```python
from build123d import *

# Parameters (mm, degrees)
SKETCH1_W           = 34
SKETCH1_H           = 17
SKETCH1_R           = 2.5
BOSS_EXTRUDE1_DEPTH = 17
SKETCH6_OUTSIDE_W   = 44.328
SKETCH6_OUTSIDE_H   = 27.328
SKETCH6_OUTSIDE_W_2 = 34
SKETCH6_OUTSIDE_H_2 = 17
SKETCH6_OUTSIDE_R   = 2.5
CUT_EXTRUDE10_DEPTH = 18
SKETCH7_OUTSIDE_W   = 27.328
SKETCH7_OUTSIDE_H   = 27.328
SKETCH7_OUTSIDE_W_2 = 17
SKETCH7_OUTSIDE_H_2 = 17
CUT_EXTRUDE11_DEPTH = 17
BOSS_EXTRUDE2_DEPTH = 17
SKETCH13_R          = 2.5
BOSS_EXTRUDE3_DEPTH = 4


with BuildPart() as part:
    # sketch1 → Boss-Extrude1 (new body)
    with BuildSketch(Plane(origin=(0, 0, 0), x_dir=(1, 0, 0), z_dir=(0, 1, 0))):
        with Locations((17, -8.5)):
            Rectangle(SKETCH1_W, SKETCH1_H)
        with Locations((8.5, -8.5)):
            Circle(SKETCH1_R, mode=Mode.SUBTRACT)
        with Locations((25.5, -8.5)):
            Circle(SKETCH1_R, mode=Mode.SUBTRACT)
    extrude(amount=BOSS_EXTRUDE1_DEPTH)

    # Sketch6 outside → Cut-Extrude10 (cut, through all)
    with BuildSketch(Plane(origin=(0, 0, 0), x_dir=(-1, 0, 0), z_dir=(0, 0, -1))):
        with Locations((-17, 8.5)):
            Rectangle(SKETCH6_OUTSIDE_W, SKETCH6_OUTSIDE_H)
        with Locations((-17, 8.5)):
            Rectangle(SKETCH6_OUTSIDE_W_2, SKETCH6_OUTSIDE_H_2, mode=Mode.SUBTRACT)
        with Locations((-25.5, 8.5)):
            Circle(SKETCH6_OUTSIDE_R)
        with Locations((-8.5, 8.5)):
            Circle(SKETCH6_OUTSIDE_R)
    extrude(amount=-CUT_EXTRUDE10_DEPTH, mode=Mode.SUBTRACT)

    # Sketch7 outside → Cut-Extrude11 (cut)
    with BuildSketch(Plane(origin=(34, 0, 0), x_dir=(0, 0, -1), z_dir=(1, 0, 0))):
        with Locations((-8.5, 8.5)):
            Rectangle(SKETCH7_OUTSIDE_W, SKETCH7_OUTSIDE_H)
        with Locations((-8.5, 8.5)):
            Rectangle(SKETCH7_OUTSIDE_W_2, SKETCH7_OUTSIDE_H_2, mode=Mode.SUBTRACT)
        Polygon((-8.5, 13.492173875), (-3.507826125, 8.5), (-8.5, 3.507826125), (-13.492173875, 8.5), align=None)
    extrude(amount=-CUT_EXTRUDE11_DEPTH, mode=Mode.SUBTRACT)


with BuildPart() as body_2:
    # Mirror6: mirrored copy
    add(part.part.mirror(Plane(origin=(0, 0, 0), x_dir=(-0.5, 0, 0.866025404), z_dir=(-0.866025404, 0, -0.5))))


with BuildPart() as part_1:
    add(part.part)

    add(body_2.part)  # Boss-Extrude2 merges body 2
    # Sketch11 → Boss-Extrude2 (add)
    with BuildSketch(Plane(origin=(0, 0, 0), x_dir=(1, 0, 0), z_dir=(0, 1, 0))):
        Polygon((-14.722431864, -8.5), (0, -17), (0, 0), align=None)
    extrude(amount=BOSS_EXTRUDE2_DEPTH)

    # Sketch13 → Boss-Extrude3 (add)
    with BuildSketch(Plane(origin=(0, 0, 0), x_dir=(1, 0, 0), z_dir=(0, 1, 0))):
        Polygon((7.152847248, 12.389094852), (-8.5, 14.722431864), (0, 0), (17, 0), align=None)
        with Locations((4.652847248, 8.058967833)):
            Circle(SKETCH13_R, mode=Mode.SUBTRACT)
    extrude(amount=BOSS_EXTRUDE3_DEPTH)


solid = part_1.part
```
Check sheet for the modelled part. Datum: model origin and axes. Units: mm. A direction names the side the tool comes from. Coordinates: 2 decimals unless noted, no trailing zeros. Write each loop counter-clockwise with the first axis right and the second up, starting at its lowest first coordinate (ties: lowest second). Pieces come first, ordered by that corner, then holes. Notation, with made-up numbers: M 20,-2.75 L 37,-2.75 A24 ccw 37,16.25 Z; hole C 52,43.25 d3. An arc over 180 degrees is marked long. Use one line per item in the form item = value.
Item 1: Set-up check for faces 4 (the face through (30.81, 6.04, 5.97)), 5 (the face through (-15.8, 8.57, -10.51)), 6 (the face through (10.885, 13.635, 7.749)), 7 (the face through (17, 10, 0)): record each of +Z, -Z, +X, -X, +Y, -Y from which the full face is reachable in a straight line by a thin tool's end or side.
Answer below:
face_4 = +X
face_5 = none
face_6 = +Y, -Y
face_7 = -Z, +X, +Y
Item 2: Sectioned sample at B-B, the plane x = 8.5. Record the cut outline in (y, z).
Answer below:
outline = M 0,-10.69 L 4,-10.69 L 4,0 L 6,0 L 6,6 L 0,6 Z; M 0,11 L 6,11 L 6,17 L 0,17 Z; M 11,0 L 17,0 L 17,6 L 11,6 Z; M 11,11 L 17,11 L 17,17 L 11,17 Z
Item 3: Sectioned sample at C-C, the plane y = 2. Record the cut outline in (x, z), and give its area (3 significant figures).
Answer below:
outline = M -31.72,-20.94 L -17,-29.44 L -8.5,-14.72 L 7.15,-12.39 L 17,0 L 34,0 L 34,17 L 0,17 L -14.72,8.5 Z; hole C -20.11,-17.83 d5; hole C -11.61,-3.11 d5; hole C 4.65,-8.06 d5; hole C 8.5,8.5 d5; hole C 25.5,8.5 d5
area = 1,390 mm^2
Item 4: Gauge pin test, flat ends, axial feed: pin 1 Ø2 at (y, z) = (10.5, -21.5) entering from +X; pin 2 Ø4 at (y, z) = (14.5, -18) entering from -X; pin 3 Ø3 at (x, y) = (-13, 3.5) entering from -Z. Record the tip position at first contact, or that the pin passes through.
Answer below:
pin_1 = -11.84
pin_2 = -31.18
pin_3 = -25.11
Item 5: Release check for a two-part mould opening along Y. For faces 1 (the face through (1, 0, -1)), 2 (the face through (-7.464, 8.381, 12.69)), 3 (the face through (-15.32, 6.04, -14.6)) record: pulls with the +Y half, pulls with the -Y half, needs draft (parallel to the pull), parting line crosses it, or undercut.
Answer below:
face_1 = pulls with the -Y half
face_2 = needs draft
face_3 = undercut
Item 6: Sectioned sample at D-D, the plane z = 5. Record the cut outline in (x, y).
Answer below:
outline = M -16.74,0 L 34,0 L 34,7.01 L 27.51,7.01 A2.5 cw 23.49,7.01 L 17,7.01 L 17,9.99 L 23.49,9.99 A2.5 cw 27.51,9.99 L 34,9.99 L 34,17 L -16.74,17 Z; hole C 8.5,8.5 d5
Item 7: Sectioned sample at A-A, the plane x = 21. Record the cut outline in (y, z).
Answer below:
outline = M 0,0 L 17,0 L 17,17 L 0,17 Z; hole M 3.51,8.5 L 8.5,3.51 L 13.49,8.5 L 8.5,13.49 Z
Item 8: Material ranges on L1, parallel to Z at x = 8.5, y = 4.5; L2, parallel to Y at x = 19, z = 11; L3, parallel to Z at x = 28.5, y = 8.25, recorded low to high. Write a range as from..to.
Answer below:
L1 = 0..6, 11..17
L2 = 0..6.01, 10.99..17
L3 = 0..3.76, 13.24..17
